Can you work these out from the drawing? Everything is in mm from the part's minimum corner. A direction names the side the tool comes from. Coordinates: 2 decimals unless noted, no trailing zeros. Loops run counter-clockwise (first coordinate to the right, second up) from the corner with the lowest first, then second, coordinate; pieces in that order, holes last.
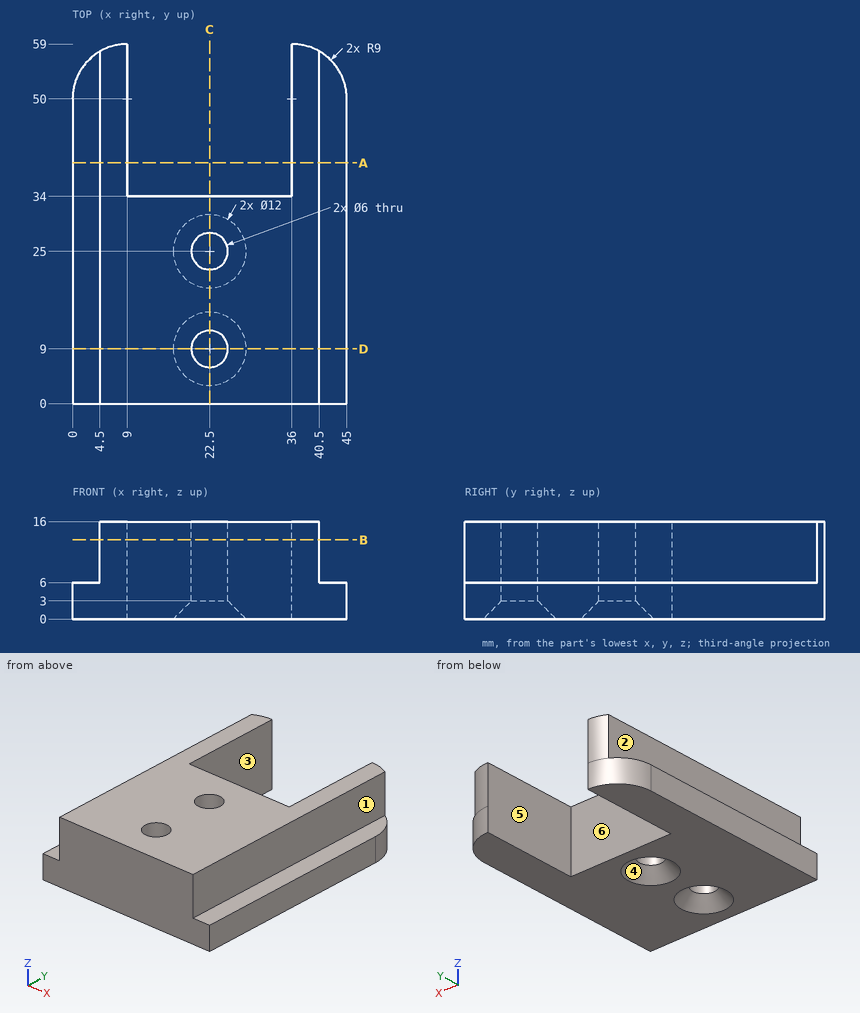
Item 1: We'd pull the mould along Y, two halves only. Please class the marked faces 4, 5 and 6: +Y half, -Y half, draft (parallel to the pull), parting line (faces both ways), or undercut.
Results are:
face 4: undercut
face 5: draft
face 6: +Y half
Item 2: Suppose I cut it at A-A, the plane y = 39.5. Please give me the cut outline in (x, z), plus the area to 3 significant figures.
Results are:
outline: (0, 0) - (9, 0) - (9, 16) - (4.5, 16) - (4.5, 6) - (0, 6) - close; (36, 0) - (45, 0) - (45, 6) - (40.5, 6) - (40.5, 16) - (36, 16) - close
area: 198 mm2
Item 3: Suppose I cut it at C-C, the plane x = 22.5. Please give me the cut outline in (y, z).
Results are:
outline: (0, 0) - (3, 0) - (6, 3) - (6, 16) - (0, 16) - close; (12, 3) - (15, 0) - (19, 0) - (22, 3) - (22, 16) - (12, 16) - close; (28, 3) - (31, 0) - (34, 0) - (34, 16) - (28, 16) - close
Item 4: Suppose I cut it at B-B, the plane z = 13. Please give me the cut outline in (x, y).
Results are:
outline: (4.5, 0) - (40.5, 0) - (40.5, 57.79) arc R9 ccw to (36, 59) - (36, 34) - (9, 34) - (9, 59) arc R9 ccw to (4.5, 57.79) - close; hole circle Ø6 at (22.5, 9); hole circle Ø6 at (22.5, 25)
Item 5: On a 3-axis mill with a long thin cutter (end or side, diameter ignored), from which of +Z, -Z, +X, -X, +Y, -Y can I reach the whole of each face in a straight line? I mean the marked faces 1, 2 and 3. Say none if no direction works.
Results are:
face 1: +Z, +X, +Y, -Y
face 2: +Z, -X, +Y, -Y
face 3: +Z, -Z, +Y
Item 6: Suppose I cut it at D-D, the plane y = 9. Please give me the cut outline in (x, z).
Results are:
outline: (0, 0) - (16.5, 0) - (19.5, 3) - (19.5, 16) - (4.5, 16) - (4.5, 6) - (0, 6) - close; (25.5, 3) - (28.5, 0) - (45, 0) - (45, 6) - (40.5, 6) - (40.5, 16) - (25.5, 16) - close
Item 7: I'm going to push flat-ended pins straight in: P1, Ø8, axis at y = 50, z = 12.5, coming from the +X side; P2, Ø7, axis at x = 22.5, y = 9, coming from the -Z side; P3, Ø5, axis at x = 19.5, z = 6, coming from the +Y side. Where does each tip first touch, or does it pass through?
Results are:
P1: stops at x = 40.5
P2: stops at z = 2.5
P3: stops at y = 34
Item 8: I need wall thicknesses on line 1 along Y through (x, z) = (22.5, 8.5); line 2 along X through (y, z) = (9, 9); line 3 along X through (y, z) = (52.5, 10). Which ranges of each line are inside material? Lowest first, please.
Results are:
line 1: y = 0 to 6, 12 to 22, 28 to 34
line 2: x = 4.5 to 19.5, 25.5 to 40.5
line 3: x = 4.5 to 9, 36 to 40.5
